from build123d import *

# Parameters (mm, degrees)
RESSALTO_EXTRUS_O1_DEPTH = 12.5
ESBO_O2_R                = 1
CORTE_EXTRUS_O1_DEPTH    = 12.5
RESSALTO_EXTRUS_O2_DEPTH = 4


with BuildPart() as part:
    # Esboço1 → Ressalto-extrusão1 (new body)
    with BuildSketch(Plane.XY):
        Polygon((-11.2, -11.4), (11.2, -11.4), (11.2, 4.7), (15.9, 4.7), (15.9, 6.7), (11.2, 6.7), (11.2, 11.4), (-11.2, 11.4), (-11.2, 6.7), (-15.9, 6.7), (-15.9, 4.7), (-11.2, 4.7), align=None)
    extrude(amount=RESSALTO_EXTRUS_O1_DEPTH)

    # Esboço2 → Corte-extrusão1 (cut)
    with BuildSketch(Plane(origin=(0, 11.4, 0), x_dir=(1, 0, 0), z_dir=(0, 1, 0))):
        with BuildLine():
            Line((-14.511437828, -7), (-15.9, -7))
            Line((-15.9, -7), (-15.9, -5.5))
            Line((-15.9, -5.5), (-14.511437828, -5.5))
            ThreePointArc((-14.511437828, -5.5), (-12.85, -6.25), (-14.511437828, -7))
        make_face()
        with Locations((13.85, -6.25)):
            Circle(ESBO_O2_R)
        with BuildLine():
            ThreePointArc((14.85, -6.25), (14.761437828, -6.661437828), (14.511437828, -7))
            Line((14.511437828, -7), (15.9, -7))
            Line((15.9, -7), (15.9, -5.5))
            Line((15.9, -5.5), (14.511437828, -5.5))
            ThreePointArc((14.511437828, -5.5), (14.761437828, -5.838562172), (14.85, -6.25))
        make_face()
    extrude(amount=-CORTE_EXTRUS_O1_DEPTH, mode=Mode.SUBTRACT)

    # Esboço3 → Ressalto-extrusão2 (add)
    with BuildSketch(Plane(origin=(0, 11.4, 0), x_dir=(1, 0, 0), z_dir=(0, 1, 0))):
        with BuildLine():
            ThreePointArc((-0.98, -8.224234029), (11.2, -6.25), (-0.98, -4.275765971))
            ThreePointArc((-0.98, -4.275765971), (-3.3, -6.25), (-0.98, -8.224234029))
        make_face()
    extrude(amount=RESSALTO_EXTRUS_O2_DEPTH)


solid = part.part
For this review, take the finished solid that the model builds, in its own axes (mm). A direction names the side the tool comes from. Round coordinates to 2 decimals unless told otherwise and drop trailing zeros. Write each loop counter-clockwise with the first axis right and the second up, starting at its lowest first coordinate (ties: lowest second). Pieces come first, ordered by that corner, then holes. Notation, with made-up numbers: M 82,34 L 138,34 A18 ccw 138,41 Z; hole C -32.5,62 d2. An arc over 180 degrees is marked long. Write item = value, one per line. Start each with the question number.
(1) The part is to be moulded in two halves that separate along X. For faces 4 (the face through (0, -11.4, 6)), 5 (the face through (12.85, 5.71, 6.22)), 6 (the face through (-11.2, -3, 6)), 7 (the face through (11.2, 9, 6)), say which applies: +X half, -X half, draft (parallel to the pull), parting line (faces both ways), or undercut.
(2) For line 1 along Z through (x, y) = (-13.85, 5.95); line 2 along X through (y, z) = (5.2, 6.25); line 3 along X through (y, z) = (-0.75, 10), list the stretches that pass through material, from the lowest coordinate up.
(3) Clearance check with flat-ended pins moving along their axes: pin 1 Ø4 at (x, z) = (-3, 4) entering from +Y; pin 2 Ø3 at (y, z) = (0, 9) entering from -X; pin 3 Ø1.6 at (x, z) = (-13.85, 6.25) entering from -Y; pin 4 Ø5 at (x, z) = (14, 6.5) entering from +Y. State where each tip first meets the part, or that it passes through.
(4) We need section D-D (x = -10). Give the boundary of the cut face in (y, z).
(5) We need section C-C (y = -9.25). Give the boundary of the cut face in (x, z).
(6) We need section A-A (x = -13.85). Give the boundary of the cut face in (y, z).
(7) For faces 1 (the face through (-15, 6, 7)), 2 (the face through (10, 11.4, 11)), 3 (the face through (-12, 6.7, 6)), list the 3-axis set-ups (+Z, -Z, +X, -X, +Y, -Y) from which the entire face can be reached by the end or side of a thin tool; tool diameter is ignored.
(8) We need section B-B (z = 2). Give the boundary of the cut face in (x, y), then the cut area to 3 significant figures.
Results found:
q1.face_4 = draft
q1.face_5 = undercut
q1.face_6 = -X half
q1.face_7 = +X half
q2.line_1 = 0 to 5.25, 7.25 to 12.5
q2.line_2 = -12.85 to 12.85
q2.line_3 = -11.2 to 11.2
q3.pin_1 = 15.4
q3.pin_2 = -11.2
q3.pin_3 = through
q3.pin_4 = 6.7
q4.outline = M -11.4,0 L 11.4,0 L 11.4,12.5 L -11.4,12.5 Z
q5.outline = M -11.2,0 L 11.2,0 L 11.2,12.5 L -11.2,12.5 Z
q6.outline = M 4.7,0 L 6.7,0 L 6.7,5.25 L 4.7,5.25 Z; M 4.7,7.25 L 6.7,7.25 L 6.7,12.5 L 4.7,12.5 Z
q7.face_1 = -X, +Y, -Y
q7.face_2 = +Z, +X, +Y
q7.face_3 = +Z, -Z, -X, +Y
q8.outline = M -15.9,4.7 L -11.2,4.7 L -11.2,-11.4 L 11.2,-11.4 L 11.2,4.7 L 15.9,4.7 L 15.9,6.7 L 11.2,6.7 L 11.2,11.4 L 9.53,11.4 L 9.53,15.4 L 0.37,15.4 L 0.37,11.4 L -11.2,11.4 L -11.2,6.7 L -15.9,6.7 Z
q8.area = 566 mm²
